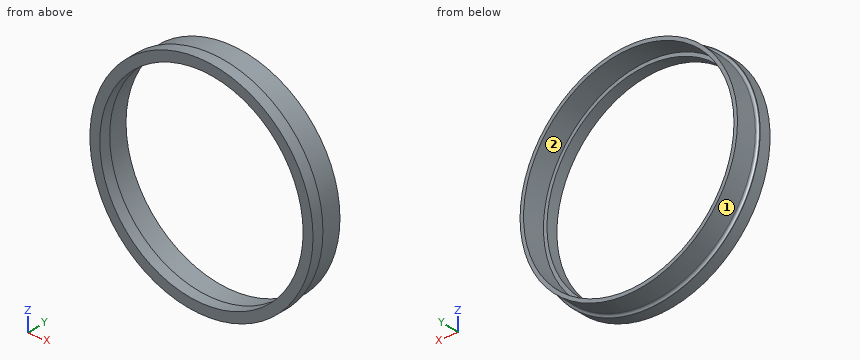
from build123d import *

# Parameters (mm, degrees)
F0_R     = 250.825
F0_R_2   = 228.6
F1_DEPTH = 76.2
F2_R     = 250.825
F2_R_2   = 244.475
F3_DEPTH = 50.8
F4_R     = 5.08
F5_R     = 236.5375
F5_R_2   = 228.6
F6_DEPTH = 50.8


with BuildPart() as f1:
    # F0 (on Front) → F1 (new body)
    with BuildSketch(Plane.XZ):
        Circle(F0_R)
        Circle(F0_R_2, mode=Mode.SUBTRACT)
    extrude(amount=F1_DEPTH)

    # F2 (on face) → F3 (cut)
    with BuildSketch(Plane(origin=(0, 0, 0), x_dir=(-1, 0, 0), z_dir=(0, 1, 0))):
        Circle(F2_R)
        Circle(F2_R_2, mode=Mode.SUBTRACT)
    extrude(amount=-F3_DEPTH, mode=Mode.SUBTRACT)

    # F4
    f4_edges = [f1.edges().sort_by_distance(p)[0] for p in [
        (244.475, -50.8, 0),
    ]]
    fillet(f4_edges, radius=F4_R)

    # F5 (on face) → F6 (cut)
    with BuildSketch(Plane(origin=(0, 0, 0), x_dir=(-1, 0, 0), z_dir=(0, 1, 0))):
        Circle(F5_R)
        Circle(F5_R_2, mode=Mode.SUBTRACT)
    extrude(amount=-F6_DEPTH, mode=Mode.SUBTRACT)


solid = f1.part
Verification items for the finished model (mm, model axes). Face numbers are marked on the shaded views. Coordinates: 2 decimals unless noted, no trailing zeros. Order: outer loops, then holes, each group sorted by start corner. A loop starts at its lowest first (then second) coordinate and runs counter-clockwise, first axis right, second up. Notation, with made-up numbers: M 78,-18 L 129,-18 A29 ccw 129,13 Z; hole C 75,-28 d9. An arc over 180 degrees is marked long. Return JSON: item names as keys, results as strings.
1) Thickness scan on L1, parallel to Z at x = 0, y = -39 (1 decimal); L2, parallel to Z at x = 0, y = -67 (3 decimals); L3, parallel to X at y = -11, z = -101. Record the ranges inside material, lowest first. Write a range as [from, to].
Answer list:
{"L1": "[-244.5, -236.5], [236.5, 244.5]", "L2": "[-250.825, -228.6], [228.6, 250.825]", "L3": "[-222.64, -213.89], [213.89, 222.64]"}
2) Release check for a two-part mould opening along X. For the marked faces 1 and 2 record: +X half, -X half, draft (parallel to the pull), parting line (faces both ways), or undercut.
Answer list:
{"face 1": "parting line", "face 2": "undercut"}
3) Cross-section at A-A, the plane x = 0. Record the boundary of the cut face in (y, z) (1 decimal), and give its area (3 significant figures).
Answer list:
{"outline": "M -76.2,-250.8 L -50.8,-250.8 L -50.8,-249.6 A5.1 cw -45.7,-244.5 L 0,-244.5 L 0,-236.5 L -50.8,-236.5 L -50.8,-228.6 L -76.2,-228.6 Z; M -76.2,228.6 L -50.8,228.6 L -50.8,236.5 L 0,236.5 L 0,244.5 L -45.7,244.5 A5.1 cw -50.8,249.6 L -50.8,250.8 L -76.2,250.8 Z", "area": "1,950 mm2"}
4) Cross-section at B-B, the plane z = 0. Record the boundary of the cut face in (x, y) (1 decimal), and give its area (3 significant figures).
Answer list:
{"outline": "M -250.8,-76.2 L -228.6,-76.2 L -228.6,-50.8 L -236.5,-50.8 L -236.5,0 L -244.5,0 L -244.5,-45.7 A5.1 cw -249.6,-50.8 L -250.8,-50.8 Z; M 228.6,-76.2 L 250.8,-76.2 L 250.8,-50.8 L 249.6,-50.8 A5.1 cw 244.5,-45.7 L 244.5,0 L 236.5,0 L 236.5,-50.8 L 228.6,-50.8 Z", "area": "1,950 mm2"}
5) Gauge pin test, flat ends, axial feed: pin 1 (1.5 mm diameter, centred on y = -46.5, z = 24.5, fed in from -X); pin 2 (12 mm diameter, centred on y = -9, z = -83.5, fed in from +X); pin 3 (10 mm diameter, centred on y = -20, z = 106.5, fed in from +X). Record the tip position at first contact, or that the pin passes through.
Answer list:
{"pin 1": "x = -243.49", "pin 2": "x = 231.87", "pin 3": "x = 222.41"}
